Autodesk Inventor part; units mm, degrees
ref_plane "YZ Plane" through (0, 0, 0) normal (1, 0, 0) x (0, 1, 0)
ref_plane "XY Plane" through (0, 0, 0) normal (0, 0, 1) x (1, 0, 0)
sketch "Sketch1" plane through (0, 0, 0) normal (0, 1, 0) x (-1, 0, 0)
  line L0 (16, 18) -> (16, -18) construction
  circle A0 centre (16, -18) radius 2
  line L1 (16, 0) -> (0, 0) construction
  line L2 (-16, 0) -> (0, 0) construction
  line L3 (-16, 18) -> (-16, -18) construction
  circle A1 centre (-16, 18) radius 2
  circle A2 centre (-16, -18) radius 2
  line L4 (22, -25.5) -> (-22, -25.5) construction
  line L5 (-22, -25.5) -> (22, -25.5)
  line L6 (-22, -25.5) -> (-22, 25.5)
  line L7 (22, -25.5) -> (-22, 25.5) construction
  line L8 (-22, -25.5) -> (22, 25.5) construction
  circle A3 centre (16, 18) radius 2
  line L9 (-22, 25.5) -> (22, 25.5) construction
  line L10 (-22, 25.5) -> (22, 25.5)
  circle A4 centre (16, -18) radius 4
  circle A5 centre (-16, -18) radius 4
  circle A6 centre (-16, 18) radius 4
  circle A7 centre (16, 18) radius 4
  line L11 (22, -25.5) -> (-22, -25.5)
  line L12 (-22, -25.5) -> (-22, -39)
  line L13 (-22, -39) -> (22, -39)
  line L14 (22, -39) -> (22, -25.5)
  line L15 (22, 25.5) -> (-22, 25.5)
  line L16 (-22, 25.5) -> (-22, 39)
  line L17 (-22, 39) -> (22, 39)
  line L18 (22, 39) -> (22, 25.5)
  line L19 (22, 0) -> (9.75, 0) construction
  line L20 (9.75, 0) -> (9.75, 10) construction
  line L21 (9.75, 0) -> (9.75, -10) construction
  line L22 (29.75, 10) -> (9.75, 10)
  line L23 (9.75, 10) -> (9.75, 14)
  line L24 (9.75, 14) -> (29.75, 14)
  line L25 (9.75, -10) -> (29.75, -10)
  line L26 (9.75, -10) -> (9.75, -14)
  line L27 (9.75, -14) -> (29.75, -14)
  line L28 (9.75, 10) -> (5.75, 10)
  line L29 (5.75, 10) -> (5.75, -10)
  line L30 (5.75, -10) -> (9.75, -10)
  line L31 (9.75, -10) -> (9.75, 10)
  line L32 (9.75, 14) -> (5.75, 14)
  line L33 (5.75, 14) -> (5.75, 10)
  line L34 (5.75, -10) -> (5.75, -14)
  line L35 (5.75, -14) -> (9.75, -14)
  line L36 (22, 0) -> (16, 0) construction
  line L37 (34.75, 46.236) -> (34.75, -49.0008) construction
  line L38 (22, 39) -> (29.75, 39)
  line L39 (29.75, 39) -> (29.75, -39)
  line L40 (29.75, -39) -> (22, -39)
  line L41 (22, 25.5) -> (22, -25.5)
  point P0 (9.75, -10)
  point P1 (9.75, 0)
  dimension "d0" = 36
  dimension "d1" = 4
  dimension "d2" = 4
  dimension "d3" = 36
  dimension "d4" = 4
  dimension "d5" = 4
  dimension "d6" = 32
  dimension "d7" = 51
  dimension "d8" = 44
  dimension "d9" = 2
  dimension "d10" = 2
  dimension "d11" = 2
  dimension "d12" = 2
  dimension "d13" = 13.5
  dimension "d14" = 13.5
  dimension "d19" = 4
  dimension "d20" = 20
  dimension "d75" = 9.75
  dimension "d79" = 20
  dimension "d80" = 34.75
extrude "Extrusion1" add sketch "Sketch1" against normal blind 4 contours L5 L14 L13 L12 | L16 L17 L18 L10
extrude "Extrusion2" add sketch "Sketch1" along normal blind 5 contours A0 | A1 | A2 | A4 | A7 | L6 L10 L41 L24 L32 L33 L29 L34 L35 L27 L5 | L5 L14 L13 L12 | L41 L27 L39 L40 L14 | L16 L17 L18 L10 | L41 L25 L39 L27 | L27 L26 L25 L41 | L18 L38 L39 L24 L41 | L41 L22 L39 L25 | L25 L31 L22 L41 | L41 L22 L23 L24 | L24 L39 L22 L41 | L35 L34 L30 L26 | L30 L29 L28 L31 | L28 L33 L32 L23 | A3 | A5 | A6
extrude "Extrusion14" add sketch "Sketch1" against normal blind 20 contours L41 L27 L39 L40 L14 | L41 L25 L39 L27 | L18 L38 L39 L24 L41 | L41 L22 L39 L25 | L24 L39 L22 L41
extrude "Extrusion3" add sketch "Sketch1" along normal blind 20 from surface at 5 contours L41 L25 L39 L27 | L27 L26 L25 L41 | L41 L22 L23 L24 | L24 L39 L22 L41 | L35 L34 L30 L26 | L30 L29 L28 L31 | L28 L33 L32 L23
extrude "Extrusion4" cut sketch "Sketch1" along normal through all contours A0 | A1 | A2 | A3
sketch "Sketch3" plane through (-9.75, 5, 10) normal (0, 0, -1) x (-1, 0, 0)
  circle A0 centre (10, 10) radius 2.2
  circle A1 centre (10, 10) radius 4.2
  line L0 (20, 0) -> (20, 20)
  line L1 (0, 0) -> (20, 0)
  dimension "d63" = 4.4
  dimension "d64" = 2
  dimension "d94" = 10
  dimension "d101" = 10
sketch "Sketch4" plane through (-29.75, -20, -39) normal (-1, 0, 0) x (0, 0, 1)
  line L0 (53, 45) -> (72.9998, 25.0002)
  line L1 (53, 45) -> (81.284, 45) construction
  line L2 (72.9998, 25.0002) -> (53, 25.0002)
  line L3 (53, 25.0002) -> (53, 45)
  point P0 (39, 20)
  dimension "d95" = 28.284
  dimension "d96" = 45
extrude "Extrusion15" cut sketch "Sketch3" against normal through all contours A0
extrude "Extrusion16" add sketch "Sketch4" against normal blind 4
extrude "Extrusion17" add sketch "Sketch4" along normal blind 4 from surface at -24
mirror "Mirror1" about plane through (0, 0, 0) normal (0, 0, 1) of "Extrusion16", "Extrusion17", "Extrusion15"
equation "\"d2\" = d1"
equation "\"d4\" = d1"
equation "\"d5\" = d1"
equation "\"d10\" = d9"
equation "\"d11\" = d9"
equation "\"d12\" = d9"
equation "\"d14\" = d13"
properties part number "XY Rail Bracket"
Could you check a few things on this model? Use its own coordinates, in mm. A direction names the side the tool comes from. Round coordinates to 2 decimals unless told otherwise and drop trailing zeros. Order: outer loops, then holes, each group sorted by start corner. A loop starts at its lowest first (then second) coordinate and runs counter-clockwise, first axis right, second up.
(1) I'm going to push flat-ended pins straight in: pin 1 (10 mm diameter, centred on y = 14, z = -23.5, fed in from +X); pin 2 (6 mm diameter, centred on y = -10.5, z = 12, fed in from +X); pin 3 (8 mm diameter, centred on x = -6.5, z = -16, fed in from -Y). Where does each tip first touch, or does it pass through?
Response values:
pin 1: stops at x = -5.75
pin 2: stops at x = -22
pin 3: stops at y = 0
(2) Which directions (+Z, -Z, +X, -X, +Y, -Y) give clear straight access to the entire face, cutting with the end or side of a thin tool? Please do faces 4 (the flat face through (-5.75, 13, 0)), 5 (the flat face through (-9.75, 11, -20)), 6 (the flat face through (0, -4, 32)), 7 (the flat face through (-22.1, 14.9, 10)).
Response values:
face 4: +Z, -Z, +X, +Y
face 5: -Z, +Y
face 6: +Z, -Z, +X, -Y
face 7: -X, +Y
(3) Please list where these lines run through material, in increasing order: line 1 along X through (y, z) = (1.95, -18); line 2 along Z through (x, y) = (5.5, -2); line 3 along Z through (x, y) = (-22, 12).
Response values:
line 1: x = -29.75 to -18, -14 to 14, 18 to 22
line 2: z = -39 to -25.5, 25.5 to 39
line 3: z = -14 to -10, 10 to 14
(4) Imagine slicing it at B-B (z = -18). Write out the boundary of the cut face in (x, y), plus the area to 3 significant figures.
Response values:
outline: (-29.75, -20) - (-22, -20) - (-22, 0) - (-18, 0) - (-18, 5) - (-29.75, 5) - close; (-29.75, 5) - (-25.75, 5) - (-25.75, 21) - (-29.75, 21) - close; (-14, 0) - (14, 0) - (14, 5) - (-14, 5) - close; (-9.75, 5) - (-5.75, 5) - (-5.75, 21) - (-9.75, 21) - close; (18, 0) - (22, 0) - (22, 5) - (18, 5) - close
area: 502 mm2
(5) If we mould it in two halves opening along X, with no side actions, what happens to faces 1 (the cylindrical face through (-16, 2, 16)), 2 (the flat face through (-9.75, 15, 0)), 3 (the flat face through (-9, -2, -39))? For each: released by +X, released by -X, zero draft, split by the parting line, or undercut.
Response values:
face 1: undercut
face 2: released by -X
face 3: zero draft
(6) Imagine slicing it at A-A (x = 16). Write out the boundary of the cut face in (y, z), plus the area to 3 significant figures.
Response values:
outline: (-4, -39) - (5, -39) - (5, -20) - (0, -20) - (0, -25.5) - (-4, -25.5) - close; (-4, 25.5) - (0, 25.5) - (0, 20) - (5, 20) - (5, 39) - (-4, 39) - close; (0, -16) - (5, -16) - (5, 16) - (0, 16) - close
area: 458 mm2
(7) Imagine slicing it at C-C (z = 22). Write out the boundary of the cut face in (x, y).
Response values:
outline: (-29.75, -20) - (-22, -20) - (-22, 0) - (22, 0) - (22, 5) - (-29.75, 5) - close; (-29.75, 5) - (-25.75, 5) - (-25.75, 17) - (-29.75, 17) - close; (-9.75, 5) - (-5.75, 5) - (-5.75, 17) - (-9.75, 17) - close
